```python
from build123d import *

# Parameters (mm, degrees)
BOSS_EXTRUDE1_DEPTH = 5.08


with BuildPart() as part:
    # Sketch1 → Boss-Extrude1 (new body)
    with BuildSketch(Plane(origin=(0, 0, 0), x_dir=(1, 0, 0), z_dir=(0, 1, 0))):
        with BuildLine():
            Line((22.225, 22.225), (22.225, 15.875))
            Line((22.225, 15.875), (12.7, 15.875))
            Line((12.7, 15.875), (12.7, 10.795))
            Line((12.7, 10.795), (22.225, 10.795))
            Line((22.225, 10.795), (22.225, 5.55625))
            Line((22.225, 5.55625), (12.7, 5.55625))
            ThreePointArc((12.7, 5.55625), (7.14375, 0), (12.7, -5.55625))
            Line((12.7, -5.55625), (22.225, -5.55625))
            Line((22.225, -5.55625), (22.225, -10.795))
            Line((22.225, -10.795), (12.7, -10.795))
            Line((12.7, -10.795), (12.7, -15.875))
            Line((12.7, -15.875), (22.225, -15.875))
            Line((22.225, -15.875), (22.225, -22.225))
            Line((22.225, -22.225), (0, -22.225))
            Line((0, -22.225), (0, 0))
            Line((0, 0), (0, 22.225))
            Line((0, 22.225), (22.225, 22.225))
        make_face()
    extrude(amount=BOSS_EXTRUDE1_DEPTH)


solid = part.part
```
Design review of the part built by this model. Coordinates are the model's own, in mm. A direction names the side the tool comes from. Coordinates: 2 decimals unless noted, no trailing zeros. Order: outer loops, then holes, each group sorted by start corner. A loop starts at its lowest first (then second) coordinate and runs counter-clockwise, first axis right, second up. Notation, with made-up numbers: (-5, 87.25) - (19, 87.25) arc R30 ccw to (19, 121.25) - close; hole circle Ø1 at (60, -13.5). An arc over 180 degrees is marked (long way). One line per question, with ' | ' between items.
Q1. Clearance check with flat-ended pins moving along their axes: pin 1 Ø2 at (y, z) = (3.5, 3) entering from +X; pin 2 Ø6 at (x, z) = (14, 17.5) entering from -Y; pin 3 Ø2.5 at (y, z) = (1.5, -14.5) entering from +X; pin 4 Ø1 at (x, z) = (9.5, 2.5) entering from -Y. State where each tip first meets the part, or that it passes through.
Answer key:
pin 1: stops at x = 8.84 | pin 2: stops at y = 0 | pin 3: stops at x = 12.7 | pin 4: passes through
Q2. Consider section B-B, the plane y = 0.6. Give the boundary of the cut face in (x, z) (1 decimal), then the cut area to 3 significant figures.
Answer key:
outline: (0, -22.2) - (22.2, -22.2) - (22.2, -15.9) - (12.7, -15.9) - (12.7, -10.8) - (22.2, -10.8) - (22.2, -5.6) - (12.7, -5.6) arc R5.6 cw to (12.7, 5.6) - (22.2, 5.6) - (22.2, 10.8) - (12.7, 10.8) - (12.7, 15.9) - (22.2, 15.9) - (22.2, 22.2) - (0, 22.2) - close | area: 737 mm2
Q3. The part is to be moulded in two halves that separate along Z. For faces 1 (the flat face through (11, 3, -22.225)), 2 (the flat face through (22.225, 3, -19)), 3 (the flat face through (12.7, 3, -13)), say which applies: +Z half, -Z half, draft (parallel to the pull), parting line (faces both ways), or undercut.
Answer key:
face 1: -Z half | face 2: draft | face 3: undercut
Q4. To check wall thickness, follow line 1 along Z through (x, y) = (17, 2.4) (3 decimals); line 2 along X through (y, z) = (2.6, -12.5); line 3 along Z through (x, y) = (8.5, 3) (3 decimals). State the ranges of each line that lie inside material, in increasing order.
Answer key:
line 1: z = -22.225 to -15.875, -10.795 to -5.556, 5.556 to 10.795, 15.875 to 22.225 | line 2: x = 0 to 12.7 | line 3: z = -22.225 to -3.638, 3.638 to 22.225
Q5. Consider section C-C, the plane z = 0. Give the boundary of the cut face in (x, y), then the cut area to 3 significant figures.
Answer key:
outline: (0, 0) - (7.14, 0) - (7.14, 5.08) - (0, 5.08) - close | area: 36.3 mm2
Q6. For faces 4 (the flat face through (11, 3, 22.225)), 5 (the flat face through (12.7, 3, 13)), list the 3-axis set-ups (+Z, -Z, +X, -X, +Y, -Y) from which the entire face can be reached by the end or side of a thin tool; tool diameter is ignored.
Answer key:
face 4: +Z, +X, -X, +Y, -Y | face 5: +X, +Y, -Y
Q7. Consider section A-A, the plane x = 18.5. Give the boundary of the cut face in (y, z) (3 decimals), then the cut area to 3 significant figures.
Answer key:
outline: (0, -22.225) - (5.08, -22.225) - (5.08, -15.875) - (0, -15.875) - close; (0, -10.795) - (5.08, -10.795) - (5.08, -5.556) - (0, -5.556) - close; (0, 5.556) - (5.08, 5.556) - (5.08, 10.795) - (0, 10.795) - close; (0, 15.875) - (5.08, 15.875) - (5.08, 22.225) - (0, 22.225) - close | area: 118 mm2
